Check sheet for the modelled part. Datum: model origin and axes. Units: mm. A direction names the side the tool comes from. Round coordinates to 2 decimals unless told otherwise and drop trailing zeros. Order: outer loops, then holes, each group sorted by start corner. A loop starts at its lowest first (then second) coordinate and runs counter-clockwise, first axis right, second up.
Q1. Scan lines: probe 1 along X at (y, z) = (2, 1); probe 2 along Y at (x, z) = (5.75, -1); probe 3 along X at (y, z) = (0.25, 1.25). Record each from-to range of solid material in increasing order.
Q2. Cross-section at A-A on x = 9.75. Record the cut outline in (y, z), then the cut area to 3 significant figures.
Q3. Set-up check for faces 1 (the flat face through (0, 2, -2)), 2 (the cylindrical face through (-1.825, 3.233, 1.341)), 3 (the flat face through (-2.948, 0.761, 1.293)): record each of +Z, -Z, +X, -X, +Y, -Y from which the full face is reachable in a straight line by a thin tool's end or side.
Q4. Depth check by flat-ended pin: P1, Ø1.5, axis at y = -2.5, z = 1.5, coming from the +X side; P2, Ø1.5, axis at x = 2, z = 1.5, coming from the +Y side; P3, Ø2, axis at x = 5.5, z = -2.5, coming from the +Y side. Enter the tip coordinate at first touch or a pass-through.
Q5. Mould release check, pull along Y, two halves, no side actions. Record for faces 4 (the flat face through (14, 0, 0)), 5 (the cylindrical face through (7, 0, 2)), 6 (the flat face through (-3, 1.5, 0)): +Y half, -Y half, draft (parallel to the pull), parting line (faces both ways), or undercut.
Autodesk Inventor part; units mm, degrees
ref_plane "Work Plane1" through (29, 0, 0) normal (0, -1, 0) x (1, 0, 0)
ref_plane "YZ Plane" through (0, 0, 0) normal (1, 0, 0) x (0, 1, 0)
ref_plane "XZ Plane" through (0, 0, 0) normal (0, 1, 0) x (-1, 0, 0)
sketch "Sketch1" plane through (0, 0, 0) normal (0, 0, 1) x (1, 0, 0)
  line L0 (-1, 0) -> (14, 0)
  line L1 (14, 0) -> (14, 2)
  line L2 (14, 2) -> (1.75, 2)
  line L3 (1.75, 2) -> (1.3205, 2)
  line L4 (1.3205, 2) -> (0, 2)
  line L5 (0, 2) -> (0, 3.5)
  line L6 (0, 3.5) -> (-4, 3.5)
  line L7 (-4, 3.5) -> (-4, 1.7321)
  line L8 (-4, 1.7321) -> (-2, 1.7321)
  line L9 (-2, 1.7321) -> (-1, 0)
  line L10 (-7.6, 0) -> (17.6, 0)
  line L11 (0, -0.7) -> (0, 4.2)
  line L12 (1.75, 2) -> (0, 2) construction
  dimension "d1" = 12.25
  dimension "d2" = 0.4295
  dimension "d3" = 4
  dimension "d4" = 2
  dimension "d5" = 60
  dimension "d6" = 4
  dimension "d7" = 4
  dimension "d8" = 3.4641
  dimension "d9" = 7
  dimension "d26" = 14
revolve "Body" add sketch "Sketch1" angle 360 about axis through (-1, 0, 0) along (1, 0, 0)
sketch "Sketch2" plane through (-4, 0, 0) normal (-1, 0, 0) x (0, 0, 1)
  circle A0 centre (0, 0) radius 1.7321
  line L0 (0, -4.9) -> (0, 4.9)
  line L1 (-4.9, 0) -> (4.9, 0)
  line L2 (1.7321, 0) -> (0.866, -1.5)
  line L3 (0.866, -1.5) -> (-0.866, -1.5)
  line L4 (-0.866, -1.5) -> (-1.7321, 0)
  line L5 (-1.7321, 0) -> (-0.866, 1.5)
  line L6 (-0.866, 1.5) -> (0.866, 1.5)
  line L7 (0.866, 1.5) -> (1.7321, 0)
extrude "Slot" add sketch "Sketch2" against normal up to next contours L7 A0 | A0 L2 | L6 L0 A0 | A0 L0 L3 | L0 L6 A0 | A0 L3 L0 | L4 A0 | A0 L5
fillet "Fillet1" radius 0.4 1 edges at (-4, -3.5, 0)
thread "Thread"
chamfer "Chamfer1" distance 0.4294 distance2 0.4294 1 edges at (14, -2, 0) measured on face at (14, 0.527, -0.2661)
ref_plane "Work Plane1" through (29, 0, 0) normal (0, -1, 0) x (1, 0, 0)
fillet "Fillet2" radius 0.1 1 edges at (0, -2, 0)
equation "\"d1\" = GEL"
equation "\"d3\" = KOH"
equation "\"d4\" = INTI"
equation "\"d6\" = GD"
equation "\"d7\" = BDM"
equation "\"d8\" = 1.1547 * SW"
equation "\"d9\" = KOD"
equation "\"d26\" = NLG"
equation "\"d30\" = R"
equation "\"d17\" = RR"
equation "\"d13\" = GEL"
equation "\"d15\" = -0.5 * SPD + 0.5 * GD"
equation "\"d16\" = GUL"
equation "\"GD\" = NND"
equation "\"NLG\" = 14"
equation "\"GEL\" = 12.25"
equation "\"KOD\" = 7"
equation "\"KOH\" = NND"
equation "\"INTI\" = 2"
equation "\"GAL\" = 0.61345 * PTC"
equation "\"GUL\" = 0.61345 * PTC"
equation "\"BDM\" = NND"
equation "\"SW\" = 3"
equation "\"RR\" = 0.1 * NND"
equation "\"SPD\" = NND - 1.2269 * PTC"
equation "\"R\" = 0.1"
equation "\"PHH\" = 0.13"
equation "\"GD1\" = THREADDIA - 1.2269 * PTC"
equation "\"THREADDIA\" = 4"
equation "\"FAWI\" = 45deg"
equation "\"PTC\" = 0.7"
equation "\"KOH1\" = 3.6"
equation "\"NND\" = 4"
equation "\"TOA\" = 30deg"
equation "\"E0\" = 1.155 * SW"
properties part number "AS 1420 - 1973 - M4 x 14" material "Steel, Mild"
Results found:
1. probe 1: x = -4 to 0
1. probe 2: y = -1.73 to 1.73
1. probe 3: x = -1.74 to 14
2. outline: circle Ø4 at (0, 0)
2. area: 12.6 mm2
3. face 1: +X
3. face 2: +X, -X
3. face 3: -X
4. P1: stops at x = 0
4. P2: stops at y = 1.85
4. P3: stops at y = 1.32
5. face 4: draft
5. face 5: parting line
5. face 6: undercut
